```python
from build123d import *

# Parameters (mm, degrees)
SKETCH1_R           = 3
BOSS_EXTRUDE1_DEPTH = 10


with BuildPart() as part:
    # Sketch1 → Boss-Extrude1 (new body)
    with BuildSketch(Plane.XY):
        with BuildLine():
            Line((-12.5, 0), (-12.5, -212.108992783))
            Line((-12.5, -212.108992783), (45, -212.108992783))
            Line((45, -212.108992783), (45, -187.108992783))
            Line((45, -187.108992783), (12.5, -187.108992783))
            Line((12.5, -187.108992783), (12.5, 0))
            ThreePointArc((12.5, 0), (0, 12.5), (-12.5, 0))
        make_face()
        Circle(SKETCH1_R, mode=Mode.SUBTRACT)
        with Locations((32.5, -199.608992783)):
            Circle(SKETCH1_R, mode=Mode.SUBTRACT)
    extrude(amount=BOSS_EXTRUDE1_DEPTH)


solid = part.part
```
Verification items for the finished model (mm, model axes). Round coordinates to 2 decimals unless told otherwise and drop trailing zeros. Order: outer loops, then holes, each group sorted by start corner. A loop starts at its lowest first (then second) coordinate and runs counter-clockwise, first axis right, second up. Notation, with made-up numbers: (-27, 76.25) - (-14, 76.25) arc R27 cw to (-14, 105.25) - close; hole circle Ø4 at (43, 37.25). An arc over 180 degrees is marked (long way). Use CSV: the item, a comma, the result in double quotes.
(1) Section check C-C on x = 32.5. Record the boundary of the cut face in (y, z).
Entries:
outline,"(-212.11, 0) - (-202.61, 0) - (-202.61, 10) - (-212.11, 10) - close; (-196.61, 0) - (-187.11, 0) - (-187.11, 10) - (-196.61, 10) - close"
(2) Section check B-B on z = 8.25. Record the boundary of the cut face in (x, y), and give its area (3 significant figures).
Entries:
outline,"(-12.5, -212.11) - (45, -212.11) - (45, -187.11) - (12.5, -187.11) - (12.5, 0) arc R12.5 ccw to (-12.5, 0) - close; hole circle Ø6 at (0, 0); hole circle Ø6 at (32.5, -199.61)"
area,"6,300 mm^2"
(3) Gauge pin test, flat ends, axial feed: pin 1 Ø2 at (x, z) = (11.5, 3) entering from +Y; pin 2 Ø3 at (x, z) = (13, 8.5) entering from +Y; pin 3 Ø9.5 at (x, y) = (0, 0) entering from +Z; pin 4 Ø4 at (x, z) = (37, 4.5) entering from +Y. Record the tip position at first contact, or that the pin passes through.
Entries:
pin 1,"y = 6.78"
pin 2,"y = 4.9"
pin 3,"z = 10"
pin 4,"y = -187.11"
(4) Section check A-A on x = 0. Record the boundary of the cut face in (y, z), and give its area (3 significant figures).
Entries:
outline,"(-212.11, 0) - (-3, 0) - (-3, 10) - (-212.11, 10) - close; (3, 0) - (12.5, 0) - (12.5, 10) - (3, 10) - close"
area,"2,190 mm^2"
(5) Mould release check, pull along X, two halves, no side actions. Record for faces 1 (the face through (-3, 0, 5)), 2 (the face through (30.119, -201.434, 4.93)), 3 (the face through (12.5, -95, 5)), 4 (the face through (29, -187.109, 5)): released by +X, released by -X, zero draft, split by the parting line, or undercut.
Entries:
face 1,"undercut"
face 2,"undercut"
face 3,"released by +X"
face 4,"zero draft"
(6) Section check D-D on y = -120.5. Record the boundary of the cut face in (x, z).
Entries:
outline,"(-12.5, 0) - (12.5, 0) - (12.5, 10) - (-12.5, 10) - close"
(7) Thickness scan on probe 1 along Y at (x, z) = (0, 9); probe 2 along Y at (x, z) = (32.5, 7.25); probe 3 along X at (y, z) = (-58, 5). Record the ranges inside material, lowest first. Write a range as from..to.
Entries:
probe 1,"-212.11..-3, 3..12.5"
probe 2,"-212.11..-202.61, -196.61..-187.11"
probe 3,"-12.5..12.5"
